Could you check a few things on this model? Use its own coordinates, in mm. A direction names the side the tool comes from. Coordinates: 2 decimals unless noted, no trailing zeros. Write each loop counter-clockwise with the first axis right and the second up, starting at its lowest first coordinate (ties: lowest second). Pieces come first, ordered by that corner, then holes.
Item 1: I want a section at D-D on y = -2.55. Please give me the cut outline in (x, z), then the cut area to 3 significant figures.
Item 2: For P1, Ø2, axis at x = 9, y = -3.5, coming from the -Z side; P2, Ø6, axis at x = 12.5, z = 14.5, coming from the -Y side; P3, Ø0.5, axis at x = -10, y = 0.5, coming from the +Z side; P4, Ø2, axis at x = 2, y = -3.5, coming from the +Z side, each with a flat end and sliding along its axis, tell me the tip position at first contact or that it passes through.
Item 3: Thinking about a two-plate mould opening in X: for faces 5 (the flat face through (-0.2, 0.5, -21)), 6 (the flat face through (10.993, 0.5, -9.5)), which applies, +X half, -X half, draft (parallel to the pull), parting line (faces both ways), or undercut?
Item 4: I want a section at B-B on z = 2. Please give me the cut outline in (x, y), then the cut area to 3 significant figures.
Item 5: If I drill on probe 1 along Y at (x, z) = (3, 9); probe 2 along X at (y, z) = (-0.3, -2.5); probe 3 along Y at (x, z) = (11.5, -3.5), over which ranges is the centre line in solid material (lowest first)?
Item 6: Which directions (+Z, -Z, +X, -X, +Y, -Y) give clear straight access to the entire face, cutting with the end or side of a thin tool? Please do faces 1 (the flat face through (10.993, 0.5, 20.5)), 2 (the cylindrical face through (6.38, -1.97, 2.65)), 3 (the flat face through (11.5, -0.5, 5)), 4 (the flat face through (8.993, 0.5, 0.5)).
Item 7: I want a section at A-A on x = 0. Please give me the cut outline in (y, z), then the cut area to 3 significant figures.
Item 8: I want a section at C-C on x = -9.5. State how many separate pieces and enclosed holes the cut face has, then the cut area to 3 significant figures.
Autodesk Fusion 360 part; units mm, degrees
sketch "Sketch1" plane through (0, 0, 0) normal (0, 1, 0) x (1, 0, 0)
  circle A0 centre (0, 0) radius 6.91
  dimension "d1" = 13.82
extrude "Extrude1" add sketch "Sketch1" against normal blind 4 makes body 1
sketch "Sketch2" plane through (0, 0, 0) normal (0, 1, 0) x (1, 0, 0)
  line L0 (11, -21) -> (-11, -21)
  line L1 (-11, -21) -> (-11, 21)
  line L2 (-11, 21) -> (11, 21)
  line L3 (11, 21) -> (11, -21)
  line L4 (11, -21) -> (-11, 21) construction
  line L5 (-11, -21) -> (11, 21) construction
  dimension "d4" = 22
  dimension "d5" = 42
extrude "Extrude2" add sketch "Sketch2" along normal blind 1 bodies 1
extrude "Extrude3" add 1 faces at (-11, 0.3333, 7) along direction (-1, 0, 0) blind 5 on bodies 1 bodies 1
extrude "Extrude4" add 1 faces at (11, 0.3333, -7) along direction (1, 0, 0) blind 5 on bodies 1 bodies 1
sketch "Sketch3" plane through (0, 0, 0) normal (0, -1, 0) x (1, 0, 0)
  line L0 (-16, -21) -> (16, -21)
  line L1 (16, -21) -> (16, 21)
  line L2 (16, 21) -> (-16, 21)
  line L3 (-16, 21) -> (-16, -21)
  circle A0 centre (0, 0) radius 6.91
  line L4 (11, -10) -> (12, -10)
  line L5 (12, -10) -> (12, 5)
  line L6 (12, 5) -> (11, 5)
  line L7 (11, 5) -> (11, -10)
  line L8 (-11, 10) -> (-12, 10)
  line L9 (-12, 10) -> (-12, -5)
  line L10 (-12, -5) -> (-11, -5)
  line L11 (-11, -5) -> (-11, 10)
  dimension "d67" = 15
extrude "Extrude5" add sketch "Sketch3" along normal blind 1 separate body contours L4 L5 L6 L7 makes body 2
extrude "Extrude6" add sketch "Sketch3" along normal blind 1 separate body contours L8 L9 L10 L11 makes body 3
combine "Combine1" operation add target body 1 tool bodies 2 3
sketch "Sketch4" plane through (0, 1, 0) normal (0, 1, 0) x (-1, 0, 0)
  line L0 (-16, -21) -> (16, -21)
  line L1 (16, -21) -> (16, 21)
  line L2 (16, 21) -> (-16, 21)
  line L3 (-16, 21) -> (-16, -21)
  line L4 (11.0067, 21) -> (9.0067, 21)
  line L5 (9.0067, 21) -> (9.0067, 20)
  line L6 (9.0067, 20) -> (11.0067, 20)
  line L7 (11.0067, 20) -> (11.0067, 21)
  line L8 (9.0067, 15) -> (11.0067, 15)
  line L9 (9.0067, 16) -> (9.0067, 15)
  line L10 (11.0067, 16) -> (9.0067, 16)
  line L11 (11.0067, 15) -> (11.0067, 16)
  line L12 (9.0067, 5) -> (11.0067, 5)
  line L13 (9.0067, 6) -> (9.0067, 5)
  line L14 (11.0067, 6) -> (9.0067, 6)
  line L15 (11.0067, 5) -> (11.0067, 6)
  line L16 (9.0067, 10) -> (11.0067, 10)
  line L17 (9.0067, 11) -> (9.0067, 10)
  line L18 (11.0067, 11) -> (9.0067, 11)
  line L19 (11.0067, 10) -> (11.0067, 11)
  line L20 (11.0067, 1) -> (9.0067, 1)
  line L21 (9.0067, 0) -> (11.0067, 0)
  line L22 (9.0067, 1) -> (9.0067, 0)
  line L23 (11.0067, 0) -> (11.0067, 1)
  line L24 (11.0067, -4) -> (9.0067, -4)
  line L25 (9.0067, -4) -> (9.0067, -5)
  line L26 (11.0067, -5) -> (11.0067, -4)
  line L27 (9.0067, -5) -> (11.0067, -5)
  line L28 (11.0067, -9) -> (9.0067, -9)
  line L29 (9.0067, -10) -> (11.0067, -10)
  line L30 (11.0067, -10) -> (11.0067, -9)
  line L31 (9.0067, -9) -> (9.0067, -10)
  line L32 (11.0067, -14) -> (9.0067, -14)
  line L33 (9.0067, -14) -> (9.0067, -15)
  line L34 (9.0067, -15) -> (11.0067, -15)
  line L35 (11.0067, -15) -> (11.0067, -14)
  line L36 (11.0067, -19) -> (9.0067, -19)
  line L37 (9.0067, -20) -> (11.0067, -20)
  line L38 (11.0067, -20) -> (11.0067, -19)
  line L39 (9.0067, -19) -> (9.0067, -20)
  line L40 (-10.9933, 21) -> (-10.9933, 20)
  line L41 (-10.9933, 20) -> (-8.9933, 20)
  line L42 (-8.9933, 20) -> (-8.9933, 21)
  line L43 (-8.9933, 21) -> (-10.9933, 21)
  line L44 (-10.9933, 16) -> (-10.9933, 15)
  line L45 (-10.9933, 15) -> (-8.9933, 15)
  line L46 (-8.9933, 16) -> (-10.9933, 16)
  line L47 (-8.9933, 15) -> (-8.9933, 16)
  line L48 (-10.9933, 10) -> (-8.9933, 10)
  line L49 (-8.9933, 11) -> (-10.9933, 11)
  line L50 (-10.9933, 11) -> (-10.9933, 10)
  line L51 (-8.9933, 10) -> (-8.9933, 11)
  line L52 (-10.9933, 6) -> (-10.9933, 5)
  line L53 (-8.9933, 6) -> (-10.9933, 6)
  line L54 (-10.9933, 5) -> (-8.9933, 5)
  line L55 (-8.9933, 5) -> (-8.9933, 6)
  line L56 (-8.9933, 0) -> (-8.9933, 1)
  line L57 (-10.9933, 0) -> (-8.9933, 0)
  line L58 (-8.9933, 1) -> (-10.9933, 1)
  line L59 (-10.9933, 1) -> (-10.9933, 0)
  line L60 (-8.9933, -4) -> (-10.9933, -4)
  line L61 (-10.9933, -4) -> (-10.9933, -5)
  line L62 (-10.9933, -5) -> (-8.9933, -5)
  line L63 (-8.9933, -5) -> (-8.9933, -4)
  line L64 (-8.9933, -9) -> (-10.9933, -9)
  line L65 (-10.9933, -10) -> (-8.9933, -10)
  line L66 (-10.9933, -9) -> (-10.9933, -10)
  line L67 (-8.9933, -10) -> (-8.9933, -9)
  line L68 (-8.9933, -14) -> (-10.9933, -14)
  line L69 (-10.9933, -14) -> (-10.9933, -15)
  line L70 (-8.9933, -15) -> (-8.9933, -14)
  line L71 (-10.9933, -15) -> (-8.9933, -15)
  line L72 (-8.9933, -19) -> (-10.9933, -19)
  line L73 (-10.9933, -19) -> (-10.9933, -20)
  line L74 (-10.9933, -20) -> (-8.9933, -20)
  line L75 (-8.9933, -20) -> (-8.9933, -19)
  dimension "d88" = 2
  dimension "d89" = 1
  dimension "d90" = 2
  dimension "d91" = 1
  dimension "d92" = 2
  dimension "d93" = 1
  dimension "d94" = 2
  dimension "d95" = 1
  dimension "d96" = 2
  dimension "d97" = 1
  dimension "d98" = 2
  dimension "d99" = 1
  dimension "d100" = 2
  dimension "d101" = 1
  dimension "d102" = 2
  dimension "d103" = 1
  dimension "d104" = 2
  dimension "d105" = 1
  dimension "d106" = 2
  dimension "d107" = 1
  dimension "d108" = 2
  dimension "d109" = 1
  dimension "d110" = 2
  dimension "d111" = 1
  dimension "d112" = 2
  dimension "d113" = 1
  dimension "d114" = 2
  dimension "d115" = 1
  dimension "d116" = 2
  dimension "d117" = 1
  dimension "d118" = 2
  dimension "d119" = 1
  dimension "d120" = 2
  dimension "d121" = 1
  dimension "d122" = 2
  dimension "d123" = 1
extrude "Extrude7" cut sketch "Sketch4" against normal blind 1 contours L2 L40 L41 L42 L43 | L2 L4 L5 L6 L7 | L8 L9 L10 L11 | L12 L13 L14 L15 | L16 L17 L18 L19 | L20 L21 L22 L23 | L24 L25 L26 L27 | L28 L29 L30 L31 | L32 L33 L34 L35 | L36 L37 L38 L39 | L44 L45 L46 L47 | L48 L49 L50 L51 | L52 L53 L54 L55 | L56 L57 L58 L59 | L60 L61 L62 L63 | L64 L65 L66 L67 | L68 L69 L70 L71 | L72 L73 L74 L75 bodies 1
Response values:
1. outline: circle Ø13.82 at (0, 0)
1. area: 150 mm2
2. P1: passes through
2. P2: stops at y = 0
2. P3: stops at z = 20
2. P4: stops at z = 6.84
3. face 5: draft
3. face 6: undercut
4. outline: (-16, 0) - (-12, 0) - (-12, -1) - (-11, -1) - (-11, 0) - (-6.61, 0) - (-6.61, -4) - (6.61, -4) - (6.61, 0) - (11, 0) - (11, -1) - (12, -1) - (12, 0) - (16, 0) - (16, 1) - (-16, 1) - close
4. area: 86.9 mm2
5. probe 1: y = 0 to 1
5. probe 2: x = -12 to -11, -6.44 to 6.44, 11 to 12
5. probe 3: y = -1 to 1
6. face 1: +Z, +Y, -Y
6. face 2: -Y
6. face 3: +Z, +X, -Y
6. face 4: +Y, -Y
7. outline: (-4, -6.91) - (0, -6.91) - (0, -21) - (1, -21) - (1, 21) - (0, 21) - (0, 6.91) - (-4, 6.91) - close
7. area: 97.3 mm2
8. separate pieces: 9
8. enclosed holes: 0
8. area: 33.0 mm2
